Here's how the part is built. I have some questions about the finished solid (model axes, mm). Give positions to 0.01 mm unless a question says otherwise; leave off trailing zeros. Loops run counter-clockwise (first coordinate to the right, second up) from the corner with the lowest first, then second, coordinate; pieces in that order, holes last. Notation, with made-up numbers: (-16.5, 29) - (32.5, 29) arc R29 ccw to (32.5, 68) - close; hole circle Ø6 at (15.5, 33.5). An arc over 180 degrees is marked (long way). Use one line per item in the form item = value.
from build123d import *

# Parameters (mm, degrees)
SKETCH2_R = 12.7
SKETCH5_R = 12.7


with BuildPart() as part:
    # Sweep1: sweep along a path in Sketch3
    with BuildLine(Plane(origin=(0, 0, 0), x_dir=(0, 0, -1), z_dir=(1, 0, 0))) as sweep1_path:
        Line((0, 0), (-457.2, 0))
        Line((-457.2, 0), (-457.2, 279.4))
        Line((-457.2, 279.4), (0, 279.4))
        Line((0, 279.4), (0, 0))
    # Sketch2 → Sweep1 (sweep)
    with BuildSketch(Plane.XY):
        Circle(SKETCH2_R)
    sweep(path=sweep1_path.line, transition=Transition.RIGHT)

    # Sweep2: sweep along a path in Sketch4
    with BuildLine(Plane(origin=(0, 0, 0), x_dir=(0, 0, -1), z_dir=(1, 0, 0))) as sweep2_path:
        Line((-142.063950703, 0), (-147.331360877, 280.791318963))
    # Sketch5 → Sweep2 (sweep)
    with BuildSketch(Plane(origin=(0, 0, 0), x_dir=(1, 0, 0), z_dir=(0, 1, 0))):
        with Locations((0, -142.063950703)):
            Circle(SKETCH5_R)
    sweep(path=sweep2_path.line)


solid = part.part
(1) If I drill on probe 1 along Y at (x, z) = (-0.25, 262); probe 2 along Z at (x, y) = (-6.75, 145.5); probe 3 along Y at (x, z) = (1.5, 214), over which ranges is the centre line in solid material (lowest first)?
Geometry says:
probe_1 = -12.7 to 12.7, 266.7 to 292.1
probe_2 = -10.76 to 10.76, 134.04 to 155.55, 446.44 to 467.96
probe_3 = -12.61 to 12.61, 266.79 to 292.01
(2) If we section it at B-B (x = 7): Give the number of separate pieces and of enclosed holes in the cut face, plus the area to 3 significant figures.
Geometry says:
separate_pieces = 1
enclosed_holes = 2
area = 36,700 mm²
(3) If we section it at A-A (z = 423): List the corners of the cut face in (x, y) for me.
Geometry says:
outline = circle Ø25.4 at (0, 0); circle Ø25.4 at (0, 279.4)
(4) Thinking about a two-plate mould opening in Z: for faces 1 (the cylindrical face through (-2.75, 141.83, 469.6)), 2 (the cylindrical face through (-2.75, 137.57, -12.4)), which applies, pulls with the +Z half, pulls with the -Z half, needs draft (parallel to the pull), parting line crosses it, or undercut?
Geometry says:
face_1 = undercut
face_2 = undercut
(5) For P1, Ø6, axis at x = -9, z = 164.5, coming from the -Y side; P2, Ø12, axis at x = -7, y = 25.5, coming from the -Z side; P3, Ø1.5, axis at x = 4, y = 45.5, coming from the +Z side, each with a flat end and sliding along its axis, tell me the tip position at first contact or that it passes through.
Geometry says:
P1 = -11.19
P2 = -12.66
P3 = 469.48
